The figure shows three views and two pictorial views of one solid part (mm, origin at its lowest corner). Answer the questions. A direction names the side the tool comes from. Round coordinates to 2 decimals unless told otherwise and drop trailing zeros. Loops run counter-clockwise (first coordinate to the right, second up) from the corner with the lowest first, then second, coordinate; pieces in that order, holes last. Notation, with made-up numbers: (67.5, 89.5) -> (95.5, 89.5) arc R14 ccw to (95.5, 115.5) -> close; hole circle Ø10 at (25, -33.5). An arc over 180 degrees is marked (long way). Write item = value, one per line. Start each with the question number.
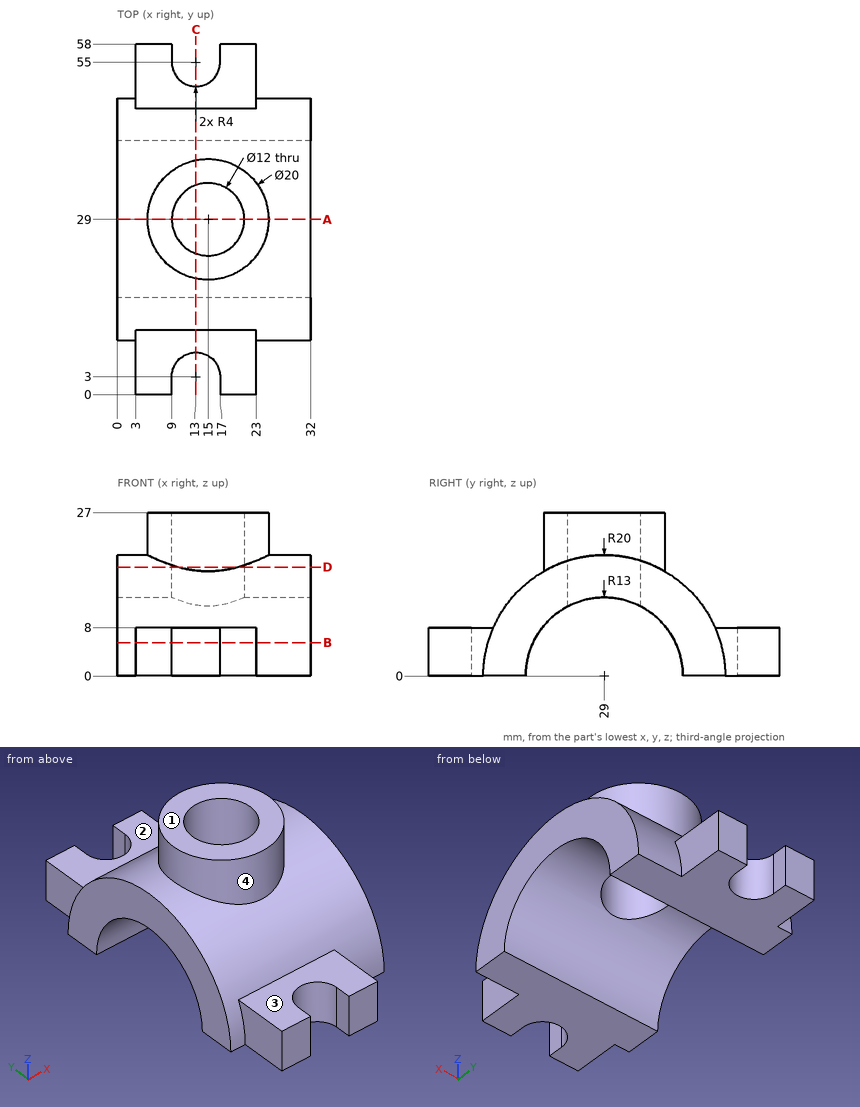
Item 1: Section C-C (x = 13) is taken. Determine the outline of the cut face in (y, z), then the cut area to 3 significant figures.
Item 2: Flat-ended cylindrical pins translate along their axes: pin 1 (3.5 mm diameter, centred on y = 56, z = 5, fed in from +X); pin 2 (5.5 mm diameter, centred on x = 16, y = 51.5, fed in from +Z); pin 3 (2.5 mm diameter, centred on y = 2.5, z = 2.5, fed in from -X). Find the tip coordinate at first contact, or state that the pin passes through.
Item 3: Section D-D (z = 18) is taken. Determine the outline of the cut face in (x, y).
Item 4: A tool of negligible diameter and unlimited length cuts with its end or side. For the marked faces 1, 2, 3 and 4, from which of +Z, -Z, +X, -X, +Y, -Y can it reach the whole face along a straight path? Write none if from no direction.
Item 5: Find the intervals of material crossed by line 1 along Y through (x, z) = (15, 17.5); line 2 along X through (y, z) = (29, 17.75); line 3 along X through (y, z) = (29, 21.5), in increasing order. Write a range as [from, to].
Item 6: Section B-B (z = 5.5) is taken. Determine the outline of the cut face in (x, y).
Item 7: Section A-A (y = 29) is taken. Determine the outline of the cut face in (x, z), then the cut area to 3 significant figures.
Worked answers:
q1.outline = (7, 0) -> (16, 0) arc R13 cw to (23.34, 11.7) -> (23.34, 27) -> (19.2, 27) -> (19.2, 17.44) arc R20 ccw to (10.67, 8) -> (7, 8) -> close; (34.66, 11.7) arc R13 cw to (42, 0) -> (51, 0) -> (51, 8) -> (47.33, 8) arc R20 ccw to (38.8, 17.44) -> (38.8, 27) -> (34.66, 27) -> close
q1.area = 394 mm2
q2.pin_1 = 23
q2.pin_2 = 8
q2.pin_3 = 3
q3.outline = (0, 20.28) -> (10.1, 20.28) arc R10 ccw to (19.9, 20.28) -> (32, 20.28) -> (32, 37.72) -> (19.9, 37.72) arc R10 ccw to (10.1, 37.72) -> (0, 37.72) -> close; hole circle Ø12 at (15, 29)
q4.face_1 = +Z, +X, -X, +Y, -Y
q4.face_2 = +Z, +X, -X, +Y
q4.face_3 = +Z, +X, -X, -Y
q4.face_4 = +Z
q5.line_1 = [19, 23], [35, 39]
q5.line_2 = [0, 9], [21, 32]
q5.line_3 = [5, 9], [21, 25]
q6.outline = (0, 9.77) -> (3, 9.77) -> (3, 0) -> (9, 0) -> (9, 3) arc R4 cw to (17, 3) -> (17, 0) -> (23, 0) -> (23, 9.77) -> (32, 9.77) -> (32, 17.22) -> (0, 17.22) -> close; (0, 40.78) -> (32, 40.78) -> (32, 48.23) -> (23, 48.23) -> (23, 58) -> (17, 58) -> (17, 55) arc R4 cw to (9, 55) -> (9, 58) -> (3, 58) -> (3, 48.23) -> (0, 48.23) -> close
q7.outline = (0, 13) -> (9, 13) -> (9, 27) -> (5, 27) -> (5, 20) -> (0, 20) -> close; (21, 13) -> (32, 13) -> (32, 20) -> (25, 20) -> (25, 27) -> (21, 27) -> close
q7.area = 196 mm2
